CAD build for the part. Positions are in the model's coordinates, mm. Face numbers are marked on the shaded views. A direction names the side the tool comes from. Give positions to 0.01 mm unless a question says otherwise; leave off trailing zeros. Write each loop counter-clockwise with the first axis right and the second up, starting at its lowest first coordinate (ties: lowest second). Pieces come first, ordered by that corner, then holes. Notation, with made-up numbers: (5.25, 12.25) -> (29.25, 12.25) arc R30 cw to (29.25, 39.25) -> close; hole circle Ø11 at (64.5, -17). An arc over 180 degrees is marked (long way). Use one line per item in the form item = value. Start each with the question number.
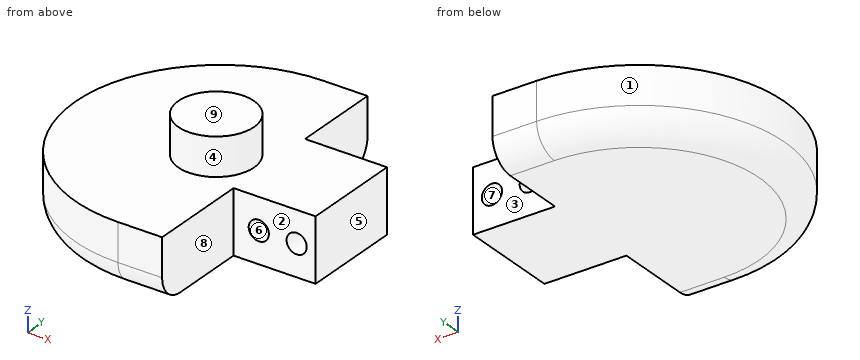
from build123d import *

# Parameters (mm, degrees)
BOSS_EXTRUDE1_DEPTH = 5
CUT_EXTRUDE1_START  = 11
SKETCH2_R           = 0.8
CUT_EXTRUDE1_DEPTH  = 23
BOSS_EXTRUDE2_START = 5
SKETCH4_R           = 3
BOSS_EXTRUDE2_DEPTH = 3
FILLET1_R           = 2


with BuildPart() as part:
    # Sketch1 → Boss-Extrude1 (new body)
    with BuildSketch(Plane.XY):
        with BuildLine():
            Line((3.5, 12), (3.5, 5))
            Line((3.5, 5), (10, 5))
            Line((10, 5), (10, -3))
            Line((10, -3), (3.5, -3))
            Line((3.5, -3), (3.5, -11))
            Line((3.5, -11), (0, -11))
            ThreePointArc((0, -11), (-11.5, 0.5), (0, 12))
            Line((0, 12), (3.5, 12))
        make_face()
    extrude(amount=BOSS_EXTRUDE1_DEPTH)

    # Sketch2 → Cut-Extrude1 (cut, through all)
    with BuildSketch(Plane(origin=(0, 0, 0), x_dir=(1, 0, 0), z_dir=(0, 1, 0)).offset(CUT_EXTRUDE1_START)):
        with Locations((8.5, -2.5)):
            Circle(SKETCH2_R)
        with Locations((5.5, -2.5)):
            Circle(SKETCH2_R)
    extrude(amount=-CUT_EXTRUDE1_DEPTH, mode=Mode.SUBTRACT)

    # Sketch4 → Boss-Extrude2 (add)
    with BuildSketch(Plane.XY.offset(BOSS_EXTRUDE2_START)):
        Circle(SKETCH4_R)
    extrude(amount=BOSS_EXTRUDE2_DEPTH)

    # Fillet1
    fillet1_edges = [part.edges().sort_by_distance(p)[0] for p in [
        (1.75, -11, 0),
        (-11.5, 0.5, 0),
        (1.75, 12, 0),
    ]]
    fillet(fillet1_edges, radius=FILLET1_R)


solid = part.part
1) Cut at D-D (z = 7). Give the cut face in (x, y), and give its area (3 significant figures).
2) Pin check, flat tips, straight feed: pin 1 (2.5 mm diameter, centred on x = 8, z = 3.5, fed in from +Y); pin 2 (1 mm diameter, centred on y = -8.5, z = 5, fed in from -X); pin 3 (1.5 mm diameter, centred on y = 8.5, z = 3, fed in from +X). Stop position of each tip, or through.
3) 3-axis set-ups, long thin cutter, end or side, ignore diameter. For the marked faces 1, 2, 3, 4 and 5: which of +Z, -Z, +X, -X, +Y, -Y reach the whole face in a straight line?
4) Cut at A-A (z = 2.5). Give the cut face in (x, y), and give its area (3 significant figures).
5) Wall check: line 1 along X through (y, z) = (0.5, 2.5); line 2 along Z through (x, y) = (8.5, 3); line 3 along X through (y, z) = (2.75, 2.5). Give the ranges that are in metal, low to high. Write a range as from..to.
6) Two-plate mould, pull along X, no slides. Class the marked faces 6, 7, 8 and 9: released by +X, released by -X, zero draft, split by the parting line, or undercut.
7) Cut at C-C (y = 0.5). Give the cut face in (x, z).
8) Cut at B-B (x = 5.5). Give the cut face in (y, z), and give its area (3 significant figures).
Final values:
q1.outline = circle Ø6 at (0, 0)
q1.area = 28.3 mm^2
q2.pin_1 = 5
q2.pin_2 = -7.75
q2.pin_3 = 3.5
q3.face_1 = +Z, -Z, -X
q3.face_2 = +Z, -Z, +X, -Y
q3.face_3 = +Z, -Z, +X, +Y
q3.face_4 = +Z
q3.face_5 = +Z, -Z, +X, +Y, -Y
q4.outline = (0, -11) -> (3.5, -11) -> (3.5, -3) -> (4.7, -3) -> (4.7, 5) -> (3.5, 5) -> (3.5, 12) -> (0, 12) arc R11.5 ccw to start; (6.3, -3) -> (7.7, -3) -> (7.7, 5) -> (6.3, 5) -> close; (9.3, -3) -> (10, -3) -> (10, 5) -> (9.3, 5) -> close
q4.area = 315 mm^2
q5.line_1 = -11.5..4.7, 6.3..7.7, 9.3..10
q5.line_2 = 0..1.7, 3.3..5
q5.line_3 = -11.28..4.7, 6.3..7.7, 9.3..10
q6.face_6 = undercut
q6.face_7 = undercut
q6.face_8 = released by +X
q6.face_9 = zero draft
q7.outline = (-11.5, 2) arc R2 ccw to (-9.5, 0) -> (10, 0) -> (10, 5) -> (2.96, 5) -> (2.96, 8) -> (-2.96, 8) -> (-2.96, 5) -> (-11.5, 5) -> close; hole circle Ø1.6 at (5.5, 2.5); hole circle Ø1.6 at (8.5, 2.5)
q8.outline = (-3, 0) -> (5, 0) -> (5, 1.7) -> (-3, 1.7) -> close; (-3, 3.3) -> (5, 3.3) -> (5, 5) -> (-3, 5) -> close
q8.area = 27.2 mm^2
